```python
from build123d import *

# Parameters (mm, degrees)
SKETCH1_R                     = 60
BOSS_EXTRUDE1_DEPTH           = 5.5
FILLET1_R                     = 2
FILLET2_R                     = 10
FILLET3_R                     = 5
FILLET4_R                     = 2.15
CSK_FOR_M4_SFHCS1_D           = 4.2
CSK_FOR_M4_SFHCS1_CSINK_D     = 10
CSK_FOR_M4_SFHCS1_CSINK_ANGLE = 90


with BuildPart() as part:
    # Sketch1 → Boss-Extrude1 (new body)
    with BuildSketch(Plane(origin=(0, 0, 0), x_dir=(1, 0, 0), z_dir=(0, 1, 0))):
        with BuildLine():
            Line((-119.071377352, -23.145131139), (-73.131225167, -14.215270156))
            ThreePointArc((-73.131225167, -14.215270156), (-58.179525881, 46.533780937), (-2.2, 74.467509694))
            Line((-2.2, 74.467509694), (-2.2, 107.4))
            Line((-2.2, 107.4), (45.8, 107.4))
            Line((45.8, 107.4), (45.8, 58.758914217))
            ThreePointArc((45.8, 58.758914217), (58.254488227, -46.439903116), (-47.074251085, -57.743093828))
            Line((-47.074251085, -57.743093828), (-109.969788273, -69.96874779))
            Line((-109.969788273, -69.96874779), (-119.071377352, -23.145131139))
        make_face()
        Circle(SKETCH1_R, mode=Mode.SUBTRACT)
    extrude(amount=BOSS_EXTRUDE1_DEPTH)

    # Fillet1
    fillet1_edges = [part.edges().sort_by_distance(p)[0] for p in [
        (-47.074251085, 2.75, 57.743093828),
    ]]
    fillet(fillet1_edges, radius=FILLET1_R)

    # Fillet2
    fillet2_edges = [part.edges().sort_by_distance(p)[0] for p in [
        (-119.071377352, 2.75, 23.145131139),
        (-2.2, 2.75, -107.4),
        (45.8, 2.75, -107.4),
        (-109.969788273, 2.75, 69.96874779),
    ]]
    fillet(fillet2_edges, radius=FILLET2_R)

    # Fillet3
    fillet3_edges = [part.edges().sort_by_distance(p)[0] for p in [
        (-73.131225167, 2.75, 14.215270156),
        (-2.2, 2.75, -74.467509694),
    ]]
    fillet(fillet3_edges, radius=FILLET3_R)

    # Fillet4
    fillet4_edges = [part.edges().sort_by_distance(p)[0] for p in [
        (45.8, 2.75, -58.758914217),
    ]]
    fillet(fillet4_edges, radius=FILLET4_R)

    # CSK for M4 SFHCS1 (through all)
    with Locations(Plane(origin=(0, 0, 0), x_dir=(-1, 0, 0), z_dir=(0, -1, 0))):
        with Locations((-22.1, 91.4), (99.767553711, -43.842048611)):
            CounterSinkHole(CSK_FOR_M4_SFHCS1_D / 2, CSK_FOR_M4_SFHCS1_CSINK_D / 2, counter_sink_angle=CSK_FOR_M4_SFHCS1_CSINK_ANGLE)


solid = part.part
```
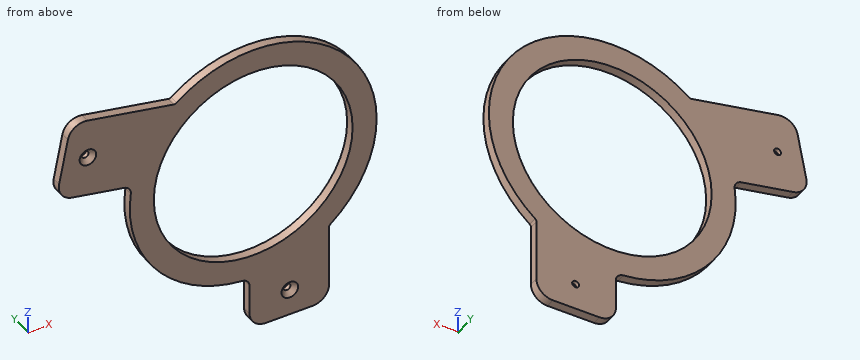
Geometry: final body of the model. Coordinates: model frame, mm. Round coordinates to 2 decimals unless told otherwise and drop trailing zeros. Order: outer loops, then holes, each group sorted by start corner. A loop starts at its lowest first (then second) coordinate and runs counter-clockwise, first axis right, second up. Notation, with made-up numbers: (3, 41) -> (8, 41) arc R19 ccw to (8, 63) -> close; hole circle Ø8 at (-2, -16). An arc over 180 degrees is marked (long way). Use one line per item in the form item = value. Start each with the question number.
1. Cut plane C-C (x = 0). Return the cut outline in (y, z).
2. Cut plane A-A (z = 6). Return the cut outline in (x, y).
3. Cut plane D-D (z = -63). Return the cut outline in (x, y).
4. Line query: probe 1 along X at (y, z) = (3.3, 0); probe 2 along X at (y, z) = (4.3, -91.4); probe 3 along Z at (x, y) = (22.1, 4). Output: solid intervals per line, ascending.
5. Pin query (flat end, axial travel): pin 1 Ø3 at (x, y) = (-87, 4.5) entering from +Z; pin 2 Ø3 at (x, z) = (-62.5, 18) entering from -Y; pin 3 Ø2 at (x, y) = (-2, 1) entering from -Z; pin 4 Ø2 at (y, z) = (2.5, 52) entering from -X. Return the tip coordinate at first contact, or that it passes through.
6. Cut plane B-B (y = 1.4). Return the cut outline in (x, z), then the cut area to 3 significant figures.
Solution:
q1.outline = (0, -103.66) -> (5.5, -103.66) -> (5.5, -60) -> (0, -60) -> close; (0, 60) -> (5.5, 60) -> (5.5, 74.5) -> (0, 74.5) -> close
q2.outline = (-74.26, 0) -> (-59.7, 0) -> (-59.7, 5.5) -> (-74.26, 5.5) -> close; (59.7, 0) -> (74.26, 0) -> (74.26, 5.5) -> (59.7, 5.5) -> close
q3.outline = (-39.76, 0) -> (45.8, 0) -> (45.8, 5.5) -> (-39.76, 5.5) -> close
q4.probe_1 = -74.5 to -60, 60 to 74.5
q4.probe_2 = -2.2 to 20, 24.2 to 45.8
q4.probe_3 = -107.4 to -93.5, -89.3 to -55.78, 55.78 to 71.15
q5.pin_1 = 65.8
q5.pin_2 = 0
q5.pin_3 = -102.15
q5.pin_4 = -113.66
q6.outline = (-117.16, 32.96) arc R10 ccw to (-109.26, 21.24) -> (-77.88, 15.14) arc R5 cw to (-73.88, 9.59) arc R74.5 ccw to (-6.75, -74.19) arc R5 cw to (-2.2, -79.17) -> (-2.2, -97.4) arc R10 ccw to (7.8, -107.4) -> (35.8, -107.4) arc R10 ccw to (45.8, -97.4) -> (45.8, -59.8) arc R2.15 cw to (46.61, -58.12) arc R74.5 ccw to (-46.36, 58.32) arc R2 cw to (-47.99, 57.92) -> (-100.15, 68.06) arc R10 ccw to (-111.88, 60.15) -> close; hole circle Ø7.2 at (-99.77, 43.84); hole circle Ø120 at (0, 0); hole circle Ø7.2 at (22.1, -91.4)
q6.area = 10,300 mm^2
